For this review, use the dimensioned drawing (mm, ordinates from the lowest corner) and the shaded views. A direction names the side the tool comes from. Coordinates: 2 decimals unless noted, no trailing zeros. Write each loop counter-clockwise with the first axis right and the second up, starting at its lowest first coordinate (ties: lowest second). Pieces come first, ordered by that corner, then holes.
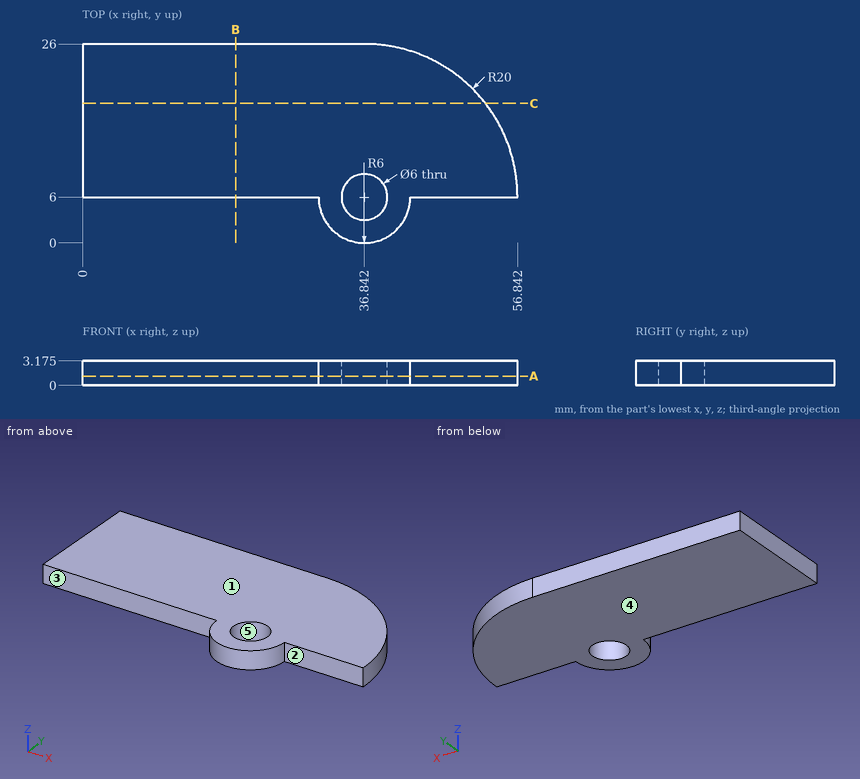
Item 1: For pin 1 (5 mm diameter, centred on x = 36.84, y = 6, fed in from -Z); pin 2 (1 mm diameter, centred on x = 12, z = 1, fed in from -Y), all flat-tipped, find the tip position at first contact; note any pin that passes through.
Solved:
pin 1: passes through
pin 2: stops at y = 6
Item 2: Take a section at B-B, the plane x = 20. Write out the cut boundary in (y, z) (3 decimals).
Solved:
outline: (6, 0) - (26, 0) - (26, 3.175) - (6, 3.175) - close
Item 3: Machinability: for the marked faces 1 and 2, which of the approach directions +Z, -Z, +X, -X, +Y, -Y give a long, thin tool a straight path to every point of the face, cutting with its end or side? Answer none if there is none.
Solved:
face 1: +Z, +X, -X, +Y, -Y
face 2: +Z, -Z, +X, -Y
Item 4: Take a section at A-A, the plane z = 1.2. Write out the cut boundary in (x, y).
Solved:
outline: (0, 6) - (30.84, 6) arc R6 ccw to (42.84, 6) - (56.84, 6) arc R20 ccw to (36.84, 26) - (0, 26) - close; hole circle Ø6 at (36.84, 6)
Item 5: To check wall thickness, follow line 1 along X through (y, z) = (4.25, 0.85) (1 decimal); line 2 along Y through (x, z) = (27, 0.9); line 3 along X through (y, z) = (6.5, 3.05). State the ranges of each line that lie inside material, in increasing order.
Solved:
line 1: x = 31.1 to 34.4, 39.3 to 42.6
line 2: y = 6 to 26
line 3: x = 0 to 33.88, 39.8 to 56.84
Item 6: Take a section at C-C, the plane y = 18.25. Write out the cut boundary in (x, z) (1 decimal).
Solved:
outline: (0, 0) - (52.7, 0) - (52.7, 3.2) - (0, 3.2) - close
Item 7: Mouldability with a two-part tool opening along Y and no side actions: class the marked faces 3, 4 and 5 as pulls with the +Y half, pulls with the -Y half, needs draft (parallel to the pull), parting line crosses it, or undercut.
Solved:
face 3: pulls with the -Y half
face 4: needs draft
face 5: undercut
